from build123d import *

# Parameters (mm, degrees)
F0_W            = 55
F0_H            = 10
F1_DEPTH        = 32.5
F3_R            = 5
F4_DEPTH        = 12.5
F6_DEPTH        = 30
F7_DEPTH        = 3
F9_D            = 3.3
F9_CSINK_D      = 6.72
F9_CSINK_ANGLE  = 90
F10_R           = 3
F11_DEPTH       = 1.5
F12_D           = 3.3
F12_DEPTH       = 13.5
F12_CSINK_D     = 6.72
F12_CSINK_ANGLE = 90
F12_TIP         = 0.9914200214
F14_D           = 2.5
F14_DEPTH       = 13.5
F14_TIP         = 0.7510757738
F16_DEPTH       = 12


# Not quite as in the source:
# - a feature names something its author has since deleted; it is built from what else it names


with BuildPart() as f1:
    # F0 (on Front) → F1 (new body, symmetric)
    with BuildSketch(Plane.XZ):
        Rectangle(F0_W, F0_H)
    extrude(amount=F1_DEPTH, both=True)

    # F3
    f3_edges = [f1.edges().sort_by_distance(p)[0] for p in [
        (27.5, -32.5, 0),
        (-27.5, -32.5, 0),
        (-27.5, 32.5, 0),
        (27.5, 32.5, 0),
    ]]
    fillet(f3_edges, radius=F3_R)

    # F2 (on Top) → F4 (cut, symmetric)
    with BuildSketch(Plane.XY):
        with BuildLine():
            ThreePointArc((-12.5, 22.5), (-16.0355339059, 21.0355339059), (-17.5, 17.5))
            Line((-17.5, 17.5), (-17.5, -30))
            Line((-17.5, -30), (17.5, -30))
            Line((17.5, -30), (17.5, 17.5))
            ThreePointArc((17.5, 17.5), (16.0355339059, 21.0355339059), (12.5, 22.5))
            Line((12.5, 22.5), (-12.5, 22.5))
        make_face()
    extrude(amount=F4_DEPTH, both=True, mode=Mode.SUBTRACT)

    # F5 (on Top) → F6 (cut)
    with BuildSketch(Plane.XY):
        with BuildLine():
            ThreePointArc((-20.75, -28.5), (-21.8106601718, -31.0606601718), (-19.25, -30))
            Line((-19.25, -30), (-20.75, -30))
            Line((-20.75, -30), (-20.75, -28.5))
        make_face()
        with BuildLine():
            ThreePointArc((-20.75, -28.5), (-19.6893398282, -28.9393398282), (-19.25, -30))
            Line((-19.25, -30), (19.25, -30))
            ThreePointArc((19.25, -30), (19.6893398282, -28.9393398282), (20.75, -28.5))
            Line((20.75, -28.5), (20.75, 28.5))
            ThreePointArc((20.75, 28.5), (19.6893398282, 28.9393398282), (19.25, 30))
            Line((19.25, 30), (-19.25, 30))
            ThreePointArc((-19.25, 30), (-19.6893398282, 28.9393398282), (-20.75, 28.5))
            Line((-20.75, 28.5), (-20.75, -28.5))
        make_face()
        with BuildLine():
            Line((-20.75, -30), (-19.25, -30))
            ThreePointArc((-19.25, -30), (-19.6893398282, -28.9393398282), (-20.75, -28.5))
            Line((-20.75, -28.5), (-20.75, -30))
        make_face()
        with BuildLine():
            ThreePointArc((20.75, -28.5), (19.6893398282, -28.9393398282), (19.25, -30))
            Line((19.25, -30), (20.75, -30))
            Line((20.75, -30), (20.75, -28.5))
        make_face()
        with BuildLine():
            Line((20.75, -30), (19.25, -30))
            ThreePointArc((19.25, -30), (20.75, -31.5), (22.25, -30))
            ThreePointArc((22.25, -30), (21.8106601718, -28.9393398282), (20.75, -28.5))
            Line((20.75, -28.5), (20.75, -30))
        make_face()
        with BuildLine():
            ThreePointArc((-19.25, 30), (-21.8106601718, 31.0606601718), (-20.75, 28.5))
            Line((-20.75, 28.5), (-20.75, 30))
            Line((-20.75, 30), (-19.25, 30))
        make_face()
        with BuildLine():
            Line((-20.75, 30), (-20.75, 28.5))
            ThreePointArc((-20.75, 28.5), (-19.6893398282, 28.9393398282), (-19.25, 30))
            Line((-19.25, 30), (-20.75, 30))
        make_face()
        with BuildLine():
            ThreePointArc((19.25, 30), (19.6893398282, 28.9393398282), (20.75, 28.5))
            Line((20.75, 28.5), (20.75, 30))
            Line((20.75, 30), (19.25, 30))
        make_face()
        with BuildLine():
            Line((20.75, 30), (20.75, 28.5))
            ThreePointArc((20.75, 28.5), (21.8106601718, 28.9393398282), (22.25, 30))
            ThreePointArc((22.25, 30), (20.75, 31.5), (19.25, 30))
            Line((19.25, 30), (20.75, 30))
        make_face()
    extrude(amount=-F6_DEPTH, mode=Mode.SUBTRACT)

    # F5 (on Top) → F7 (cut)
    with BuildSketch(Plane.XY):
        with BuildLine():
            ThreePointArc((-20.75, -28.5), (-21.8106601718, -31.0606601718), (-19.25, -30))
            Line((-19.25, -30), (-20.75, -30))
            Line((-20.75, -30), (-20.75, -28.5))
        make_face()
        with BuildLine():
            ThreePointArc((-20.75, -28.5), (-19.6893398282, -28.9393398282), (-19.25, -30))
            Line((-19.25, -30), (19.25, -30))
            ThreePointArc((19.25, -30), (19.6893398282, -28.9393398282), (20.75, -28.5))
            Line((20.75, -28.5), (20.75, 28.5))
            ThreePointArc((20.75, 28.5), (19.6893398282, 28.9393398282), (19.25, 30))
            Line((19.25, 30), (-19.25, 30))
            ThreePointArc((-19.25, 30), (-19.6893398282, 28.9393398282), (-20.75, 28.5))
            Line((-20.75, 28.5), (-20.75, -28.5))
        make_face()
        with BuildLine():
            Line((-20.75, -30), (-19.25, -30))
            ThreePointArc((-19.25, -30), (-19.6893398282, -28.9393398282), (-20.75, -28.5))
            Line((-20.75, -28.5), (-20.75, -30))
        make_face()
        with BuildLine():
            ThreePointArc((20.75, -28.5), (19.6893398282, -28.9393398282), (19.25, -30))
            Line((19.25, -30), (20.75, -30))
            Line((20.75, -30), (20.75, -28.5))
        make_face()
        with BuildLine():
            Line((20.75, -30), (19.25, -30))
            ThreePointArc((19.25, -30), (20.75, -31.5), (22.25, -30))
            ThreePointArc((22.25, -30), (21.8106601718, -28.9393398282), (20.75, -28.5))
            Line((20.75, -28.5), (20.75, -30))
        make_face()
        with BuildLine():
            ThreePointArc((-19.25, 30), (-21.8106601718, 31.0606601718), (-20.75, 28.5))
            Line((-20.75, 28.5), (-20.75, 30))
            Line((-20.75, 30), (-19.25, 30))
        make_face()
        with BuildLine():
            Line((-20.75, 30), (-20.75, 28.5))
            ThreePointArc((-20.75, 28.5), (-19.6893398282, 28.9393398282), (-19.25, 30))
            Line((-19.25, 30), (-20.75, 30))
        make_face()
        with BuildLine():
            ThreePointArc((19.25, 30), (19.6893398282, 28.9393398282), (20.75, 28.5))
            Line((20.75, 28.5), (20.75, 30))
            Line((20.75, 30), (19.25, 30))
        make_face()
        with BuildLine():
            Line((20.75, 30), (20.75, 28.5))
            ThreePointArc((20.75, 28.5), (21.8106601718, 28.9393398282), (22.25, 30))
            ThreePointArc((22.25, 30), (20.75, 31.5), (19.25, 30))
            Line((19.25, 30), (20.75, 30))
        make_face()
    extrude(amount=F7_DEPTH, mode=Mode.SUBTRACT)

    # F9 (through all)
    with Locations(Plane(origin=(0, 0, 3), x_dir=(1, 0, 0), z_dir=(0, 0, -1))):
        with Locations((-8.5, -26.5042820722), (8.5, -26.5042820722)):
            CounterSinkHole(F9_D / 2, F9_CSINK_D / 2, counter_sink_angle=F9_CSINK_ANGLE)

    # F10 (on face) → F11 (join)
    with BuildSketch(Plane.XY.offset(5)):
        with Locations((8.5, 26.5042820722)):
            Circle(F10_R)
        with Locations((-8.5, 26.5042820722)):
            Circle(F10_R)
    extrude(amount=F11_DEPTH)

    # F12
    with Locations(Plane(origin=(0, 0, 3), x_dir=(1, 0, 0), z_dir=(0, 0, -1))):
        with Locations((-8.5, -26.5042820722), (8.5, -26.5042820722)):
            CounterSinkHole(F12_D / 2, F12_CSINK_D / 2, depth=F12_DEPTH, counter_sink_angle=F12_CSINK_ANGLE)
            with Locations((0, 0, -(F12_DEPTH + F12_TIP / 2))):  # 118° drill point
                Cone(0, F12_D / 2, F12_TIP, mode=Mode.SUBTRACT)

    # F14
    with Locations(Plane(origin=(0, 0, -5), x_dir=(1, 0, 0), z_dir=(0, 0, -1))):
        with Locations((-24.125, 0), (24.125, 0), (-24.125, 17.5), (24.125, 17.5)):
            Hole(F14_D / 2, depth=F14_DEPTH)
            with Locations((0, 0, -(F14_DEPTH + F14_TIP / 2))):  # 118° drill point
                Cone(0, F14_D / 2, F14_TIP, mode=Mode.SUBTRACT)

    # F15 (on face) → F16 (cut)
    with BuildSketch(Plane(origin=(-27.5, 0, 0), x_dir=(0, -1, 0), z_dir=(-1, 0, 0))):
        with BuildLine():
            Line((-23.0304132, -5), (-10.906057547, -5))
            ThreePointArc((-10.906057547, -5), (-16.9682353735, -1.5), (-23.0304132, -5))
        make_face()
    extrude(amount=-F16_DEPTH, mode=Mode.SUBTRACT)


solid = f1.part
Geometry check sheet. Reference: the model listing, model coordinates, mm. A direction names the side the tool comes from. Round coordinates to 2 decimals unless told otherwise and drop trailing zeros. Order: outer loops, then holes, each group sorted by start corner. A loop starts at its lowest first (then second) coordinate and runs counter-clockwise, first axis right, second up. Notation, with made-up numbers: M 12,81 L 23,81 A13 ccw 23,85 Z; hole C -31,32 d2. An arc over 180 degrees is marked long. Write each question's results on one line, items separated by ' | '. Start each with the question number.
1. Cross-section at A-A on y = -17.5. Record the boundary of the cut face in (x, z) (3 decimals), plus the area to 3 significant figures.
2. Cross-section at C-C on x = -8.5. Record the boundary of the cut face in (y, z).
3. Cross-section at B-B on x = 4. Record the boundary of the cut face in (y, z), plus the area to 3 significant figures.
4. Draft check along Y on faces 5 (the face through (0, 22.5, 4)), 6 (the face through (-6.887, 29.034, 5.74)), 7 (the face through (18, 0, 5)), 8 (the face through (-21.775, 31.095, -0.944)). Enter one of: pulls with the +Y half, pulls with the -Y half, needs draft (parallel to the pull), parting line crosses it, or undercut.
5. Go/stop test with flat-tipped pins: P1, Ø22.5, axis at x = 9, y = -4, coming from the -Z side; P2, Ø2, axis at x = -24.125, y = -17.5, coming from the -Z side; P3, Ø3.5, axis at x = 20.75, y = 30, coming from the +Z side. Record where each tip stops, or that it passes through.
6. Set-up check for faces 1 (the face through (-7, 25, 6.5)), 2 (the face through (-24.2, 16.9, -1.5)), 3 (the face through (-17.5, -6, 4)), 4 (the face through (-20.75, 0, -1)): record each of +Z, -Z, +X, -X, +Y, -Y from which the full face is reachable in a straight line by a thin tool's end or side.
7. Cross-section at D-D on z = 0.75. Record the boundary of the cut face in (x, y) (3 decimals).
8. Material ranges on L1, parallel to X at y = -5, z = -2.25; L2, parallel to Y at x = 0.5, z = 4; L3, parallel to Y at x = -9.5, z = 1, recorded low to high. Write a range as from..to.
Resolved:
1) outline: M -27.5,-5 L -25.375,-5 L -25.375,5 L -27.5,5 Z; M -22.875,-5 L -20.75,-5 L -20.75,3 L -17.5,3 L -17.5,5 L -22.875,5 Z; M 17.5,3 L 20.75,3 L 20.75,-5 L 22.875,-5 L 22.875,5 L 17.5,5 Z; M 25.375,-5 L 27.5,-5 L 27.5,5 L 25.375,5 Z | area: 98.0 mm2
2) outline: M -32.5,-5 L -30,-5 L -30,5 L -32.5,5 Z; M 22.5,3 L 23.14,3 L 24.85,4.71 L 24.85,6.5 L 23.5,6.5 L 23.5,5 L 22.5,5 Z; M 28.15,4.71 L 29.86,3 L 30,3 L 30,-5 L 32.5,-5 L 32.5,5 L 29.5,5 L 29.5,6.5 L 28.15,6.5 Z
3) outline: M -32.5,-5 L -30,-5 L -30,5 L -32.5,5 Z; M 22.5,3 L 30,3 L 30,-5 L 32.5,-5 L 32.5,5 L 22.5,5 Z | area: 65.0 mm2
4) face 5: undercut | face 6: parting line crosses it | face 7: needs draft | face 8: undercut
5) P1: z = 3 | P2: through | P3: z = 5
6) face 1: +Z, +X, -X, +Y, -Y | face 2: -Z, -X | face 3: +Z, -Z | face 4: -Z
7) outline: M -27.5,-27.5 A5 ccw -22.5,-32.5 L 22.5,-32.5 A5 ccw 27.5,-27.5 L 27.5,27.5 A5 ccw 22.5,32.5 L -22.5,32.5 A5 ccw -27.5,27.5 Z; hole C -24.125,-17.5 d2.5; hole C -24.125,0 d2.5; hole M -20.75,-28.5 A1.5 ccw long -19.25,-30 L 19.25,-30 A1.5 ccw long 20.75,-28.5 L 20.75,28.5 A1.5 ccw long 19.25,30 L -19.25,30 A1.5 ccw long -20.75,28.5 Z; hole C 24.125,-17.5 d2.5; hole C 24.125,0 d2.5
8) L1: -27.5..-20.75, 20.75..27.5 | L2: -32.5..-30, 22.5..32.5 | L3: -32.5..-30, 30..32.5
